Verification items for the finished model (mm, model axes). A direction names the side the tool comes from. Coordinates: 2 decimals unless noted, no trailing zeros. Order: outer loops, then holes, each group sorted by start corner. A loop starts at its lowest first (then second) coordinate and runs counter-clockwise, first axis right, second up. Notation, with made-up numbers: M -4.5,16.25 L 39.5,16.25 A26 ccw 39.5,49.25 Z; hole C 19,-5 d6. An arc over 180 degrees is marked long. Write item = value, one per line.
```python
from build123d import *

# Parameters (mm, degrees)
BOSS_EXTRUDE1_DEPTH     = 25.4
CUT_EXTRUDE1_DEPTH      = 58.873030474
F_3_8_CLEARANCE_HOLE1_D = 10.0838
SKETCH7_W               = 4.7625
SKETCH7_H               = 19.05
BOSS_EXTRUDE2_DEPTH     = 12.7


with BuildPart() as part:
    # Sketch1 → Boss-Extrude1 (new body)
    with BuildSketch(Plane.XY):
        Polygon((-11.1125, 0), (11.1125, 0), (11.1125, 50.8), (6.35, 50.8), (6.35, 31.75), (-6.35, 31.75), (-6.35, 50.8), (-11.1125, 50.8), align=None)
    extrude(amount=BOSS_EXTRUDE1_DEPTH)

    # Sketch2 → Cut-Extrude1 (cut, through all)
    with BuildSketch(Plane.XY.offset(25.4)):
        Polygon((3.702835951, 15.9385), (-3.702835951, 15.9385), (-7.405671903, 9.525), (-3.702835951, 3.1115), (3.702835951, 3.1115), (7.405671903, 9.525), align=None)
    extrude(amount=-CUT_EXTRUDE1_DEPTH, mode=Mode.SUBTRACT)

    # 3/8 Clearance Hole1 (through all)
    with Locations(Plane.ZY.offset(11.1125)):
        with Locations((12.7, 41.275)):
            Hole(F_3_8_CLEARANCE_HOLE1_D / 2)

    # Sketch7 → Boss-Extrude2 (add)
    with BuildSketch(Plane(origin=(0, 0, 0), x_dir=(-1, 0, 0), z_dir=(0, 0, -1))):
        with Locations((-8.73125, 41.275)):
            Rectangle(SKETCH7_W, SKETCH7_H)
        with Locations((8.73125, 41.275)):
            Rectangle(SKETCH7_W, SKETCH7_H)
    extrude(amount=BOSS_EXTRUDE2_DEPTH)


solid = part.part
```
Item 1: Scan lines: L1, parallel to Y at x = 7.55, z = 12.7; L2, parallel to Y at x = 2.5, z = 7; L3, parallel to X at y = 46, z = -5. Record each from-to range of solid material in increasing order. Write a range as from..to.
Report:
L1 = 0..36.23, 46.32..50.8
L2 = 0..3.11, 15.94..31.75
L3 = -11.11..-6.35, 6.35..11.11
Item 2: Release check for a two-part mould opening along Y. For faces 1 (the flat face through (9, 31.75, -6)), 2 (the flat face through (-5.528, 12.777, 12.878)), 3 (the flat face through (9, 41, -12.7)), 4 (the flat face through (0, 15.938, 13)) record: pulls with the +Y half, pulls with the -Y half, needs draft (parallel to the pull), parting line crosses it, or undercut.
Report:
face_1 = pulls with the -Y half
face_2 = undercut
face_3 = needs draft
face_4 = undercut
Item 3: Sectioned sample at D-D, the plane x = -9.5. Enter the section's corners in (y, z) (3 decimals).
Report:
outline = M 0,0 L 31.75,0 L 31.75,-12.7 L 50.8,-12.7 L 50.8,25.4 L 0,25.4 Z; hole C 41.275,12.7 d10.084
Item 4: Gauge pin test, flat ends, axial feed: pin 1 (10 mm diameter, centred on x = -3.5, z = 6.5, fed in from -Y); pin 2 (4 mm diameter, centred on x = -7.5, z = -9.5, fed in from -Y); pin 3 (8 mm diameter, centred on x = 0, z = 12, fed in from +Y); pin 4 (3 mm diameter, centred on x = -2.5, y = 29.5, fed in from -Z). Record the tip position at first contact, or that the pin passes through.
Report:
pin_1 = 0
pin_2 = 31.75
pin_3 = 31.75
pin_4 = 0
Item 5: Sectioned sample at B-B, the plane z = -10. Enter the section's corners in (x, y), then the cut area to 3 significant figures.
Report:
outline = M -11.11,31.75 L -6.35,31.75 L -6.35,50.8 L -11.11,50.8 Z; M 6.35,31.75 L 11.11,31.75 L 11.11,50.8 L 6.35,50.8 Z
area = 181 mm^2
Item 6: Sectioned sample at A-A, the plane z = 12.7. Give the number of separate pieces and of enclosed holes in the cut face, then the cut area to 3 significant figures.
Report:
separate_pieces = 3
enclosed_holes = 1
area = 649 mm^2
Item 7: Tool access check on faces 5 (the flat face through (-0.2, 16.1, 0)), 6 (the flat face through (5.58, 12.69, 12.88)), 7 (the flat face through (-6.35, 41, 6)). Record the directions out of +Z, -Z, +X, -X, +Y, -Y that give a thin tool (end or side, any length) a straight path to the whole face; none if there is none.
Report:
face_5 = -Z, +X, -X, -Y
face_6 = +Z, -Z
face_7 = +Z, -Z, +Y
Item 8: Sectioned sample at C-C, the plane x = 4.75. Enter the section's corners in (y, z), then the cut area to 3 significant figures.
Report:
outline = M 0,0 L 4.93,0 L 4.93,25.4 L 0,25.4 Z; M 14.12,0 L 31.75,0 L 31.75,25.4 L 14.12,25.4 Z
area = 573 mm^2
